Geometry: see drawing. Coordinates: mm, zero at the bounding-box minimum. Coordinates: 2 decimals unless noted, no trailing zeros. Write each loop counter-clockwise with the first axis right and the second up, starting at its lowest first coordinate (ties: lowest second). Pieces come first, ordered by that corner, then holes.
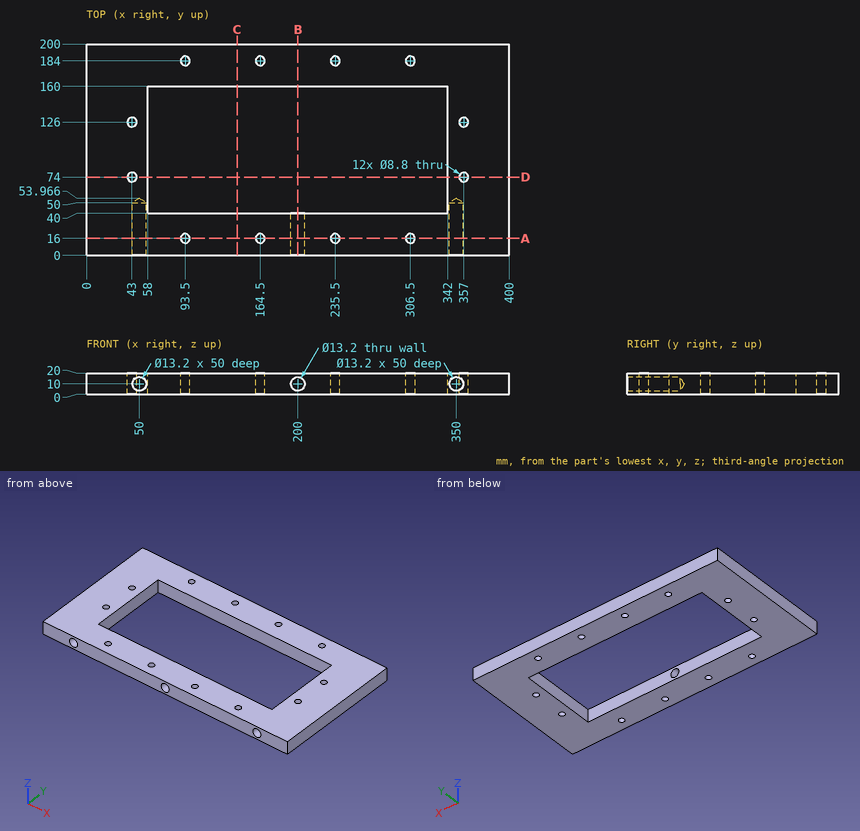
Item 1: Section A-A, the plane y = 16. Output: boundary loops of the cut face in (x, z).
Derived:
outline: (0, 0) - (89.1, 0) - (89.1, 20) - (0, 20) - close; (97.9, 0) - (160.1, 0) - (160.1, 20) - (97.9, 20) - close; (168.9, 0) - (231.1, 0) - (231.1, 20) - (168.9, 20) - close; (239.9, 0) - (302.1, 0) - (302.1, 20) - (239.9, 20) - close; (310.9, 0) - (400, 0) - (400, 20) - (310.9, 20) - close; hole circle Ø13.2 at (50, 10); hole circle Ø13.2 at (200, 10); hole circle Ø13.2 at (350, 10)
Item 2: Section D-D, the plane y = 74. Output: boundary loops of the cut face in (x, z), plus the area to 3 significant figures.
Derived:
outline: (0, 0) - (38.6, 0) - (38.6, 20) - (0, 20) - close; (47.4, 0) - (58, 0) - (58, 20) - (47.4, 20) - close; (342, 0) - (352.6, 0) - (352.6, 20) - (342, 20) - close; (361.4, 0) - (400, 0) - (400, 20) - (361.4, 20) - close
area: 1,970 mm2
Item 3: Material intervals for probe 1 along Y at (x, z) = (235.5, 9.25); probe 2 along Y at (x, z) = (357, 10.5); probe 3 along X at (y, z) = (183.5, 19), sorted ascending.
Derived:
probe 1: y = 0 to 11.6, 20.4 to 40, 160 to 179.6, 188.4 to 200
probe 2: y = 0 to 69.6, 78.4 to 121.6, 130.4 to 200
probe 3: x = 0 to 89.13, 97.87 to 160.13, 168.87 to 231.13, 239.87 to 302.13, 310.87 to 400
Item 4: Section C-C, the plane x = 142.5. Output: boundary loops of the cut face in (y, z).
Derived:
outline: (0, 0) - (40, 0) - (40, 20) - (0, 20) - close; (160, 0) - (200, 0) - (200, 20) - (160, 20) - close
Item 5: Section B-B, the plane x = 200. Output: boundary loops of the cut face in (y, z), plus the area to 3 significant figures.
Derived:
outline: (0, 0) - (40, 0) - (40, 3.4) - (0, 3.4) - close; (0, 16.6) - (40, 16.6) - (40, 20) - (0, 20) - close; (160, 0) - (200, 0) - (200, 20) - (160, 20) - close
area: 1,070 mm2
Item 6: Pin query (flat end, axial travel): pin 1 (2 mm diameter, centred on x = 50.5, z = 12, fed in from -Y); pin 2 (8 mm diameter, centred on x = 350, z = 10, fed in from -Y). Return the tip coordinate at first contact, or that it passes through.
Derived:
pin 1: stops at y = 52.13
pin 2: stops at y = 51.56
